Can you work these out from the model? Positions are in its coordinate system, mm. Face numbers are marked on the shaded views. A direction names the side the tool comes from. Coordinates: 2 decimals unless noted, no trailing zeros. Order: outer loops, then holes, each group sorted by start corner. A loop starts at its lowest first (then second) coordinate and runs counter-clockwise, first axis right, second up. Notation, with made-up numbers: (-36, 5) - (-4, 5) arc R14 ccw to (-4, 31) - close; hole circle Ø9 at (-4.75, 48). An arc over 180 degrees is marked (long way). Return JSON: item names as keys, results as strings. Group by question number.
1) For pin 1 Ø1 at (x, y) = (5.5, -0.5) entering from -Z; pin 2 Ø2 at (x, z) = (0, 7.5) entering from +Y, each with a flat end and sliding along its axis, tell me the tip position at first contact or that it passes through.
2) Imagine slicing it at B-B (y = 6.5). Write out the boundary of the cut face in (x, z).
3) Which directions (+Z, -Z, +X, -X, +Y, -Y) give clear straight access to the entire face, cutting with the end or side of a thin tool? Please do the marked faces 1, 2, 3 and 4.
4) Imagine slicing it at A-A (z = 10). Write out the boundary of the cut face in (x, y), and give its area (3 significant figures).
5) If I drill on line 1 along Z through (x, y) = (-9.5, 2.5); line 2 along Y through (x, z) = (0, 6); line 3 along Z through (x, y) = (3.25, 1.5), over which ranges is the centre line in solid material (lowest first)?
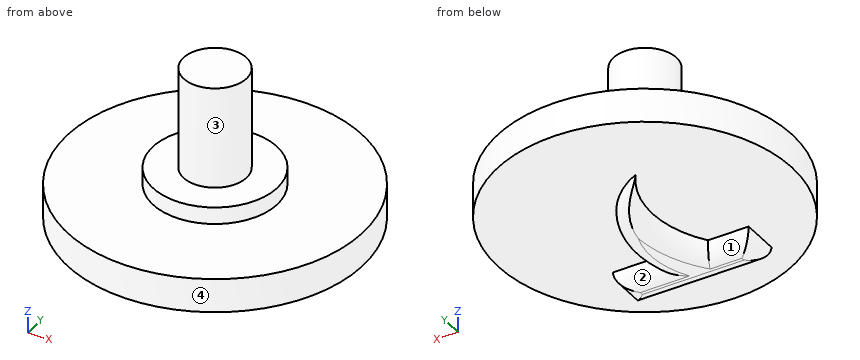
```python
from build123d import *

# Parameters (mm, degrees)
F0_R     = 2.35
F1_DEPTH = 11.43
F0_R_2   = 4.636
F2_DEPTH = 3.81
F0_R_3   = 11
F3_DEPTH = 2.54
F5_DEPTH = 1.27
F6_R     = 1.26999


# Not quite as in the source:
# - a fillet or chamfer is up to 0.001 mm smaller than in the source, because OpenCascade refuses the exact size


with BuildPart() as f1:
    # F0 (on Top) → F1 (new body)
    with BuildSketch(Plane.XY):
        Circle(F0_R)
    extrude(amount=F1_DEPTH)

    # F0 (on Top) → F2 (join)
    with BuildSketch(Plane.XY):
        Circle(F0_R_2)
        Circle(F0_R, mode=Mode.SUBTRACT)
    extrude(amount=F2_DEPTH)

    # F0 (on Top) → F3 (join)
    with BuildSketch(Plane.XY):
        Circle(F0_R_3)
        Circle(F0_R_2, mode=Mode.SUBTRACT)
    extrude(amount=F3_DEPTH)

    # F4 (on face) → F5 (join)
    with BuildSketch(Plane.XY):
        with BuildLine():
            Line((-5.0818, -4.396), (-5.0818, -7.19))
            Line((-5.0818, -7.19), (5.0782, -7.19))
            Line((5.0782, -7.19), (5.0782, -4.396))
            Line((5.0782, -4.396), (2.0302, -4.396))
            ThreePointArc((2.0302, -4.396), (1.611480541, 0.7864996759), (-2.0338, 4.494))
            ThreePointArc((-2.0338, 4.494), (-0.603014409, 0.049), (-2.0338, -4.396))
            Line((-2.0338, -4.396), (-5.0818, -4.396))
        make_face()
    extrude(amount=-F5_DEPTH)

    # F6 (radius 1.27 in the source; OpenCascade refuses exactly that, so slightly less here)
    f6_edges = [f1.edges().sort_by_distance(p)[0] for p in [
        (5.0782, -5.793, -1.27),
        (-5.0818, -5.793, -1.27),
        (-0.0018, -7.19, -1.27),
        (-3.5578, -4.396, -1.27),
        (3.5542, -4.396, -1.27),
        (1.611481, 0.7865, -1.27),
        (-0.603014, 0.049, -1.27),
    ]]
    fillet(f6_edges, radius=F6_R)


solid = f1.part
```
Calculated:
{
 "1": {"pin 1": "z = 0", "pin 2": "y = 2.35"},
 "2": {"outline": "(-8.87, 0) - (8.87, 0) - (8.87, 2.54) - (-8.87, 2.54) - close"},
 "3": {"face 1": "-Z, -X, +Y", "face 2": "-Z, +X", "face 3": "+Z", "face 4": "+Z, -Z"},
 "4": {"outline": "circle Ø4.7 at (0, 0)", "area": "17.3 mm2"},
 "5": {"line 1": "0 to 2.54", "line 2": "-2.35 to 2.35", "line 3": "0 to 3.81"}
}
